Input: part model. Units: mm. Frame: model coordinates. Face numbers are marked on the shaded views. A direction names the side the tool comes from. Coordinates: 2 decimals unless noted, no trailing zeros. Write each loop counter-clockwise with the first axis right and the second up, starting at its lowest first coordinate (ties: lowest second). Pieces come first, ordered by that corner, then holes.
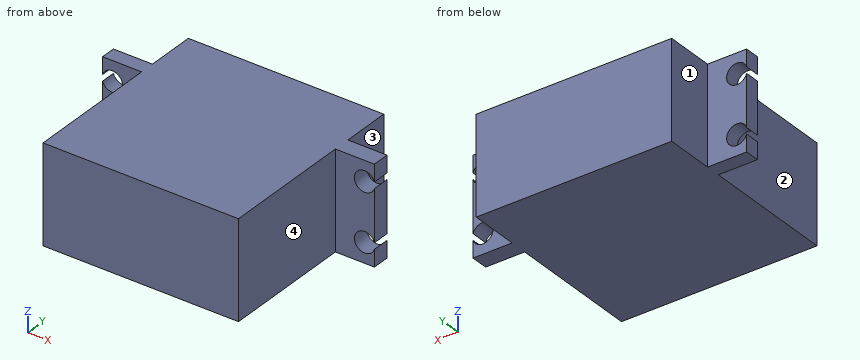
from build123d import *

# Parameters (mm, degrees)
SKETCH2_W           = 40
SKETCH2_H           = 40.5
BOSS_EXTRUDE1_DEPTH = 20
SKETCH3_W           = 20
SKETCH3_H           = 3.5
BOSS_EXTRUDE2_DEPTH = 8
SKETCH4_R           = 2.1
CUT_EXTRUDE1_DEPTH  = 8
SKETCH5_W           = 20
SKETCH5_H           = 3
BOSS_EXTRUDE3_DEPTH = 8
SKETCH6_R           = 2.1
CUT_EXTRUDE2_DEPTH  = 8


with BuildPart() as part:
    # Sketch2 → Boss-Extrude1 (new body)
    with BuildSketch(Plane.XY):
        with Locations((20, 20.25)):
            Rectangle(SKETCH2_W, SKETCH2_H)
    extrude(amount=-BOSS_EXTRUDE1_DEPTH)

    # Sketch3 → Boss-Extrude2 (add)
    with BuildSketch(Plane(origin=(40, 0, 0), x_dir=(0, 0, -1), z_dir=(1, 0, 0))):
        with Locations((10, 28.75)):
            Rectangle(SKETCH3_W, SKETCH3_H)
    extrude(amount=BOSS_EXTRUDE2_DEPTH)

    # Sketch4 → Cut-Extrude1 (cut)
    with BuildSketch(Plane(origin=(0, 30.5, 0), x_dir=(1, 0, 0), z_dir=(0, 1, 0))):
        with Locations((46, 15.9)):
            Circle(SKETCH4_R)
        with Locations((46, 4.1)):
            Circle(SKETCH4_R)
    extrude(amount=-CUT_EXTRUDE1_DEPTH, mode=Mode.SUBTRACT)

    # Sketch5 → Boss-Extrude3 (add)
    with BuildSketch(Plane.ZY):
        with Locations((-10, 29)):
            Rectangle(SKETCH5_W, SKETCH5_H)
    extrude(amount=BOSS_EXTRUDE3_DEPTH)

    # Sketch6 → Cut-Extrude2 (cut)
    with BuildSketch(Plane(origin=(0, 30.5, 0), x_dir=(1, 0, 0), z_dir=(0, 1, 0))):
        with Locations((-6, 15.9)):
            Circle(SKETCH6_R)
        with Locations((-6, 4.1)):
            Circle(SKETCH6_R)
    extrude(amount=-CUT_EXTRUDE2_DEPTH, mode=Mode.SUBTRACT)


solid = part.part
Item 1: Material intervals for line 1 (Z direction, x = -6, y = 29.55); line 2 (X direction, y = 5, z = -12); line 3 (X direction, y = 29.25, z = -15.9), sorted ascending.
Item 2: Section query C-C, the plane y = 33. Return loops of the section in (x, z), then the cut area to 3 significant figures.
Item 3: Section query B-B, the plane z = -4.1. Return loops of the section in (x, y).
Item 4: Section query D-D, the plane z = -10. Return loops of the section in (x, y).
Item 5: Section query A-A, the plane x = -6. Return loops of the section in (y, z), then the cut area to 3 significant figures.
Item 6: Access query for the marked faces 1, 2, 3 and 4. Directions: +Z, -Z, +X, -X, +Y, -Y. A direction counts if a zero-diameter tool reaches every point of the face in a straight line with its end or side. Return the directions, or none.
Item 7: Pin query (flat end, axial travel): pin 1 Ø5.5 at (x, z) = (-6, -4.1) entering from +Y; pin 2 Ø4 at (y, z) = (14, -7) entering from -X; pin 3 Ø2.5 at (x, z) = (43.5, -11) entering from -Y. Return the tip coordinate at first contact, or that it passes through.
The answers:
1. line 1: z = -20 to -18, -13.8 to -6.2, -2 to 0
1. line 2: x = 0 to 40
1. line 3: x = -3.9 to 43.9
2. outline: (0, -20) - (40, -20) - (40, 0) - (0, 0) - close
2. area: 800 mm2
3. outline: (-3.9, 27.5) - (0, 27.5) - (0, 0) - (40, 0) - (40, 27) - (43.9, 27) - (43.9, 30.5) - (40, 30.5) - (40, 40.5) - (0, 40.5) - (0, 30.5) - (-3.9, 30.5) - close
4. outline: (-8, 27.5) - (0, 27.5) - (0, 0) - (40, 0) - (40, 27) - (48, 27) - (48, 30.5) - (40, 30.5) - (40, 40.5) - (0, 40.5) - (0, 30.5) - (-8, 30.5) - close
5. outline: (27.5, -20) - (30.5, -20) - (30.5, -18) - (27.5, -18) - close; (27.5, -13.8) - (30.5, -13.8) - (30.5, -6.2) - (27.5, -6.2) - close; (27.5, -2) - (30.5, -2) - (30.5, 0) - (27.5, 0) - close
5. area: 34.8 mm2
6. face 1: +Z, -Z, -X, +Y
6. face 2: +Z, -Z, -X, -Y
6. face 3: +Z, -Z, +X, +Y
6. face 4: +Z, -Z, +X, -Y
7. pin 1: stops at y = 30.5
7. pin 2: stops at x = 0
7. pin 3: stops at y = 27
